Source: CAD feature listing. Evaluate the final solid. Frame: model axes, mm. A direction names the side the tool comes from. Coordinates: 2 decimals unless noted, no trailing zeros. Order: outer loops, then holes, each group sorted by start corner. A loop starts at its lowest first (then second) coordinate and runs counter-clockwise, first axis right, second up.
Autodesk Inventor part; units mm, degrees
ref_plane "YZ Plane" through (0, 0, 0) normal (1, 0, 0) x (0, 1, 0)
ref_plane "XZ Plane" through (0, 0, 0) normal (0, 1, 0) x (-1, 0, 0)
ref_plane "XY Plane" through (0, 0, 0) normal (0, 0, 1) x (1, 0, 0)
sketch "Boceto1" plane through (0, 0, 0) normal (1, 0, 0) x (0, 1, 0)
  line L0 (0.7564, 13.5) -> (-0.2436, 13.5)
  line L1 (-0.2436, 13.5) -> (-0.2436, -13.5)
  line L2 (-0.2436, -13.5) -> (0.7564, -13.5)
  line L3 (0.7564, -13.5) -> (0.7564, 13.5)
  point P0 (0, 0)
  dimension "d0" = 1
  dimension "d1" = 27
  dimension "d2" = 13.5
extrude "Extrusión1" add sketch "Boceto1" along normal blind 64.47
sketch "Boceto2" plane through (0, -0.2436, -13.5) normal (0, -1, 0) x (1, 0, 0)
  line L0 (0, 0) -> (64.47, 0)
  line L1 (0, 27) -> (0, 0)
  line L2 (0, 27) -> (0, 0)
  line L3 (0, 0) -> (64.47, 0)
  line L4 (64.47, 27) -> (64.47, 0)
  line L5 (0, 27) -> (64.47, 27)
  line L6 (0, 13.5) -> (64.47, 13.5)
  line L7 (64.47, 0) -> (64.47, 27)
  point P0 (2.56, 3.44)
  point P1 (6.1, 3.44)
  point P2 (8.64, 3.44)
  point P3 (16.26, 3.44)
  point P4 (18.8, 3.44)
  point P5 (21.34, 3.44)
  point P6 (23.88, 3.44)
  point P7 (26.42, 3.44)
  point P8 (28.96, 3.44)
  point P9 (31.5, 3.44)
  point P10 (34.04, 3.44)
  point P11 (11.18, 3.44)
  point P12 (13.72, 3.44)
  point P13 (2.56, 23.56)
  point P14 (6.1, 23.56)
  point P15 (8.64, 23.56)
  point P16 (16.26, 23.56)
  point P17 (18.8, 23.56)
  point P18 (21.34, 23.56)
  point P19 (23.88, 23.56)
  point P20 (26.42, 23.56)
  point P21 (28.96, 23.56)
  point P22 (31.5, 23.56)
  point P23 (34.04, 23.56)
  point P24 (11.18, 23.56)
  point P25 (13.72, 23.56)
  dimension "d5" = 3.44
  dimension "d6" = 2.56
  dimension "d8" = 2.54
  dimension "d9" = 2.54
  dimension "d10" = 2.54
  dimension "d11" = 2.54
  dimension "d12" = 2.54
  dimension "d13" = 2.54
  dimension "d14" = 2.54
  dimension "d15" = 2.54
  dimension "d16" = 2.54
  dimension "d17" = 2.54
  dimension "d18" = 2.54
  dimension "d19" = 3.54
hole "Agujero1" at (2.56, -0.2436, -10.06) at (6.1, -0.2436, -10.06) at (8.64, -0.2436, -10.06) at (16.26, -0.2436, -10.06) at (18.8, -0.2436, -10.06) at (21.34, -0.2436, -10.06) at (23.88, -0.2436, -10.06) at (26.42, -0.2436, -10.06) at (28.96, -0.2436, -10.06) at (31.5, -0.2436, -10.06) at (34.04, -0.2436, -10.06) at (11.18, -0.2436, -10.06) at (13.72, -0.2436, -10.06) at (34.04, -0.2436, 10.06) at (31.5, -0.2436, 10.06) at (28.96, -0.2436, 10.06) at (26.42, -0.2436, 10.06) at (23.88, -0.2436, 10.06) at (21.34, -0.2436, 10.06) at (18.8, -0.2436, 10.06) at (16.26, -0.2436, 10.06) at (13.72, -0.2436, 10.06) at (11.18, -0.2436, 10.06) at (8.64, -0.2436, 10.06) at (6.1, -0.2436, 10.06) at (2.56, -0.2436, 10.06) direction (0, 1, 0) diameter 0.9 end through all
sketch "Boceto3" plane through (0, -0.2436, -13.5) normal (0, -1, 0) x (1, 0, 0)
  circle A0 centre (2.56, 3.44) radius 0.45
  point P0 (0, 13.5)
  point P1 (2.1371, 23.7139)
hole "Agujero2" at (2.56, -0.2436, -10.06) at (2.1371, -0.2436, 10.2139) direction (0, 1, 0) diameter 2 end through all
sketch "Boceto4" plane through (0, -0.2436, -13.5) normal (0, -1, 0) x (1, 0, 0)
  point P0 (0, 13.5)
ref_plane "Plano de trabajo1" through (0, -0.2436, -13.5) normal (0, -1, 0) x (1, 0, 0)
ref_plane "Plano de trabajo5" through (0, -0.2436, 11.183) normal (0, 0, 1) x (1, 0, 0)
ref_plane "Plano de trabajo6" through (64.47, 0.7564, -11.183) normal (0, 0, -1) x (-1, 0, 0)
sketch "Boceto5" plane through (0, 0.7564, 13.5) normal (0, 1, 0) x (1, 0, 0)
  line L0 (1.1898, 7.974) -> (1.1898, 18.6346) construction
  line L1 (1.1898, 18.6346) -> (4.3663, 18.6346) construction
  line L2 (4.3663, 18.6346) -> (4.3663, 7.974) construction
  line L3 (4.3663, 7.974) -> (1.1898, 7.974) construction
  line L4 (6.1, 5.127) -> (36.0028, 5.127)
  line L5 (36.0028, 5.127) -> (36.0028, 22.4329)
  line L6 (36.0028, 22.4329) -> (6.1, 22.4329)
  line L7 (6.1, 22.4329) -> (6.1, 5.127)
  point P0 (0, 13.5)
extrude "Extrusión2" add sketch "Boceto5" along normal blind 2
sketch "Boceto6" plane through (0, 0.7564, 13.5) normal (0, 1, 0) x (1, 0, 0)
  line L0 (1.1904, 8.2396) -> (1.1904, 18.9001) construction
  line L1 (1.1904, 18.9001) -> (4.3668, 18.9001) construction
  line L2 (4.3668, 18.9001) -> (4.3668, 8.2396) construction
  line L3 (4.3668, 8.2396) -> (1.1904, 8.2396) construction
  point P0 (0, 13.5)
sketch "Boceto7" plane through (0, -0.2436, -13.5) normal (0, -1, 0) x (1, 0, 0)
  line L0 (0, 27) -> (64.47, 27)
  line L1 (64.47, 27) -> (64.47, 0)
  line L2 (62.97, 14) -> (61.97, 14)
  line L3 (61.97, 14) -> (61.97, 13)
  line L4 (61.97, 13) -> (62.97, 13)
  line L5 (62.97, 13) -> (62.97, 14)
  point P0 (0, 13.5)
  point P1 (62.47, 13.5)
  dimension "d43" = 13.5
  dimension "d44" = 2
  dimension "d45" = 1
  dimension "d46" = 1
  dimension "d47" = 0.5
  dimension "d48" = 0.5
extrude "Extrusión3" add sketch "Boceto7" along normal blind 0.2
properties part number "lora32Placa"
Q1. Material intervals for line 1 along Z through (x, y) = (13.72, 0.55); line 2 along Z through (x, y) = (21, 1); line 3 along Y through (x, z) = (54.5, 2), sorted ascending.
Solutions:
line 1: z = -13.5 to -10.51, -9.61 to 9.61, 10.51 to 13.5
line 2: z = -8.93 to 8.37
line 3: y = -0.24 to 0.76
Q2. Section query A-A on z = -6.5. Output: boundary loops of the cut face in (x, y), plus the area to 3 significant figures.
Solutions:
outline: (0, -0.24) - (64.47, -0.24) - (64.47, 0.76) - (36, 0.76) - (36, 2.76) - (6.1, 2.76) - (6.1, 0.76) - (0, 0.76) - close
area: 124 mm2
Q3. Set-up query: faces 4 (the flat face through (21, 2, 8.373)), 5 (the cylindrical face through (2.093, 0.263, 11.213)), 6 (the flat face through (6.1, 2, 0)). Return all of +Z, -Z, +X, -X, +Y, -Y with unobstructed straight access to the full face (end or side cutting, diameter ignored); none if empty.
Solutions:
face 4: +Z, +X, -X, +Y
face 5: +Y, -Y
face 6: +Z, -Z, -X, +Y
Q4. Pin query (flat end, axial travel): P1, Ø1.6, axis at x = 2.56, z = -10.06, coming from the -Y side; P2, Ø2.5, axis at x = 2.14, z = 10.21, coming from the -Y side; P3, Ø0.6, axis at x = 22, y = 2, coming from the +Z side; P4, Ø1.6, axis at y = 2, z = 0, coming from the -X side. Return the tip coordinate at first contact, or that it passes through.
Solutions:
P1: passes through
P2: stops at y = -0.24
P3: stops at z = 8.37
P4: stops at x = 6.1
Q5. Pull-direction query (Z, two-part tool) for faces 1 (the flat face through (21, 2, -8.933)), 2 (the flat face through (36.003, 2, 0)), 3 (the cylindrical face through (3.45, 0.26, -10.52)); classes: pulls with the +Z half, pulls with the -Z half, needs draft (parallel to the pull), parting line crosses it, or undercut.
Solutions:
face 1: pulls with the -Z half
face 2: needs draft
face 3: undercut
Q6. Section query B-B on x = 7.5. Output: boundary loops of the cut face in (y, z).
Solutions:
outline: (-0.24, -13.5) - (0.76, -13.5) - (0.76, -8.93) - (2.76, -8.93) - (2.76, 8.37) - (0.76, 8.37) - (0.76, 13.5) - (-0.24, 13.5) - close
Q7. Section query C-C on x = 54. Output: boundary loops of the cut face in (y, z).
Solutions:
outline: (-0.24, -13.5) - (0.76, -13.5) - (0.76, 13.5) - (-0.24, 13.5) - close
